Drawing for the job (mm, zero at the part's lowest x, y, z). A direction names the side the tool comes from. Give positions to 0.01 mm unless a question says otherwise; leave off trailing zeros. Write each loop counter-clockwise with the first axis right and the second up, starting at its lowest first coordinate (ties: lowest second). Pieces come first, ordered by that corner, then holes. Notation, with made-up numbers: (13.5, 82) - (72.5, 82) arc R15 cw to (72.5, 110) - close; hole circle Ø7 at (28.5, -17.75). An arc over 180 degrees is marked (long way). Use CSV: the item, a comma, the result in double quotes.
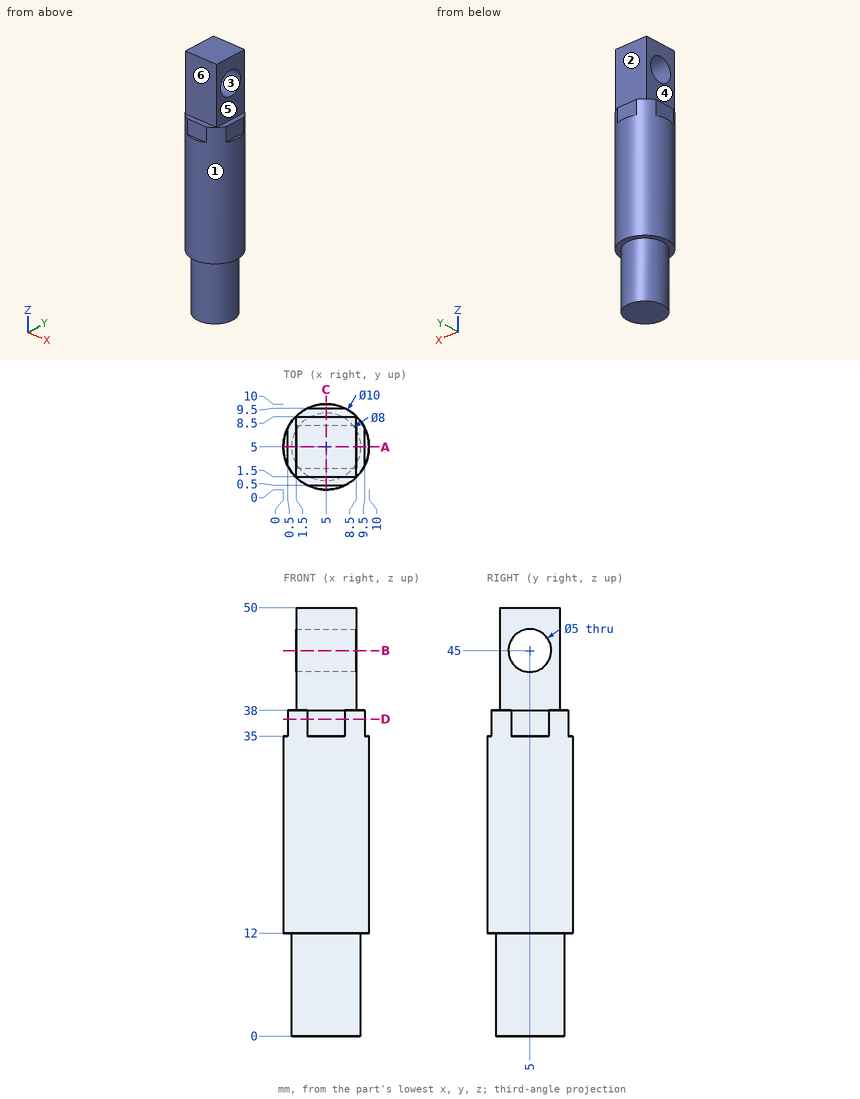
(1) Wall check: probe 1 along Y at (x, z) = (4.25, 45); probe 2 along X at (y, z) = (6.5, 37); probe 3 along Z at (x, y) = (2, 2.25). Give the ranges that are in metal, low to high. Write a range as [from, to].
Checked values:
probe 1,"y = [1.5, 2.5], [7.5, 8.5]"
probe 2,"x = [0.5, 9.5]"
probe 3,"z = [12, 50]"
(2) Saw through at C-C, the plane x = 5. List the corners of the cut face in (y, z), then the cut area to 3 significant figures.
Checked values:
outline,"(0, 12) - (1, 12) - (1, 0) - (9, 0) - (9, 12) - (10, 12) - (10, 35) - (9.5, 35) - (9.5, 38) - (8.5, 38) - (8.5, 50) - (1.5, 50) - (1.5, 38) - (0.5, 38) - (0.5, 35) - (0, 35) - close; hole circle Ø5 at (5, 45)"
area,"417 mm^2"
(3) Saw through at D-D, the plane z = 37. List the corners of the cut face in (x, y), then the cut area to 3 significant figures.
Checked values:
outline,"(0.5, 2.82) arc R5 ccw to (2.82, 0.5) - (7.18, 0.5) arc R5 ccw to (9.5, 2.82) - (9.5, 7.18) arc R5 ccw to (7.18, 9.5) - (2.82, 9.5) arc R5 ccw to (0.5, 7.18) - close"
area,"72.7 mm^2"
(4) Saw through at B-B, the plane z = 45. List the corners of the cut face in (x, y).
Checked values:
outline,"(1.5, 1.5) - (8.5, 1.5) - (8.5, 2.5) - (1.5, 2.5) - close; (1.5, 7.5) - (8.5, 7.5) - (8.5, 8.5) - (1.5, 8.5) - close"
(5) Flat gauge pins, fed straight in: P1, Ø2.5, axis at x = 4.5, z = 37, coming from the +Y side; P2, Ø1.5, axis at y = 6, z = 36, coming from the +X side; P3, Ø5.5, axis at y = 3.5, z = 45.5, coming from the -X side. Where does each tip first touch, or does it go through?
Checked values:
P1,"stops at y = 9.5"
P2,"stops at x = 9.5"
P3,"stops at x = 1.5"
(6) Pull direction Y, two halves, no side cores. Call the marked faces 1, 2 and 3: released by +Y, released by -Y, zero draft, split by the parting line, or undercut.
Checked values:
face 1,"split by the parting line"
face 2,"released by +Y"
face 3,"undercut"
(7) Saw through at A-A, the plane y = 5. List the corners of the cut face in (x, z).
Checked values:
outline,"(0, 12) - (1, 12) - (1, 0) - (9, 0) - (9, 12) - (10, 12) - (10, 35) - (9.5, 35) - (9.5, 38) - (8.5, 38) - (8.5, 42.5) - (1.5, 42.5) - (1.5, 38) - (0.5, 38) - (0.5, 35) - (0, 35) - close; (1.5, 47.5) - (8.5, 47.5) - (8.5, 50) - (1.5, 50) - close"
(8) 3-axis set-ups, long thin cutter, end or side, ignore diameter. For the marked faces 4, 5 and 6: which of +Z, -Z, +X, -X, +Y, -Y reach the whole face in a straight line?
Checked values:
face 4,"+Z, -X, +Y, -Y"
face 5,"+Z, +X, +Y, -Y"
face 6,"+Z, +X, -X, -Y"
